The figure shows three views and two pictorial views of one solid part (mm, origin at its lowest corner). Answer the questions. A direction names the side the tool comes from. Round coordinates to 2 decimals unless told otherwise and drop trailing zeros. Loops run counter-clockwise (first coordinate to the right, second up) from the corner with the lowest first, then second, coordinate; pieces in that order, holes last. Notation, with made-up numbers: (-30.5, 12) -> (20.5, 12) arc R25 cw to (20.5, 45) -> close; hole circle Ø11 at (16, 30.5). An arc over 180 degrees is marked (long way). Put each result on its own line as item: value.
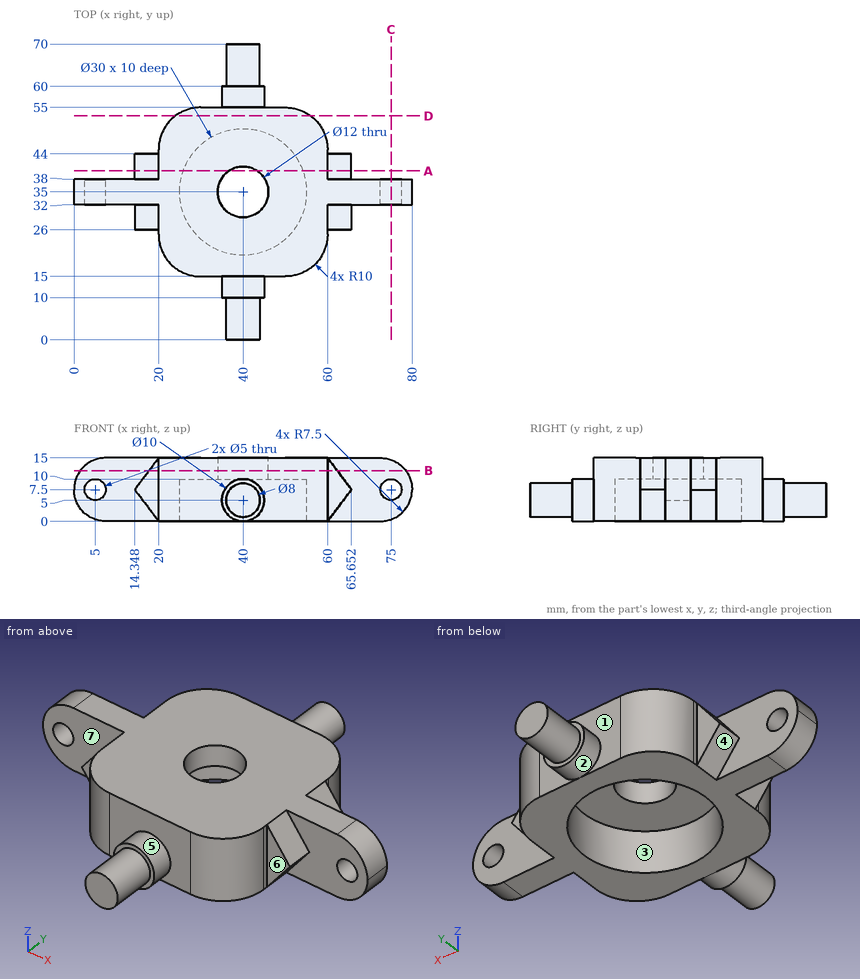
Item 1: The part is cut by section B-B (z = 12). Determine the outline of the cut face in (x, y).
Derived:
outline: (1.5, 32) -> (17.74, 32) -> (17.74, 26) -> (20, 26) -> (20, 25) arc R10 ccw to (30, 15) -> (50, 15) arc R10 ccw to (60, 25) -> (60, 26) -> (62.26, 26) -> (62.26, 32) -> (78.5, 32) -> (78.5, 38) -> (62.26, 38) -> (62.26, 44) -> (60, 44) -> (60, 45) arc R10 ccw to (50, 55) -> (30, 55) arc R10 ccw to (20, 45) -> (20, 44) -> (17.74, 44) -> (17.74, 38) -> (1.5, 38) -> close; hole circle Ø12 at (40, 35)
Item 2: The part is cut by section A-A (y = 40). Determine the outline of the cut face in (x, z).
Derived:
outline: (14.35, 7.5) -> (20, 0) -> (25.86, 0) -> (25.86, 10) -> (36.68, 10) -> (36.68, 15) -> (20, 15) -> close; (43.32, 10) -> (54.14, 10) -> (54.14, 0) -> (60, 0) -> (65.65, 7.5) -> (60, 15) -> (43.32, 15) -> close
Item 3: Which of the six approach directions +Z, -Z, +X, -X, +Y, -Y give full straight-line access (tool end or side, diameter ignored) to the marked faces 4, 5, 6 and 7?
Derived:
face 4: -Z, -X, +Y
face 5: -Y
face 6: +Z, -Z, +X, -Y
face 7: -X, -Y
Item 4: Flat-ended cylindrical pins translate along their axes: pin 1 Ø6 at (x, z) = (47.5, 5.5) entering from -Y; pin 2 Ø5 at (y, z) = (13.5, 9) entering from +X; pin 3 Ø10 at (x, y) = (38, 61) entering from -Z; pin 4 Ø3 at (x, z) = (18, 11) entering from +Y. Find the tip coordinate at first contact, or state that the pin passes through.
Derived:
pin 1: stops at y = 10
pin 2: stops at x = 54.36
pin 3: stops at z = 0
pin 4: stops at y = 44
Item 5: For a pull along Y with two mould halves and no side action, classify the marked faces 1, 2 and 3 as pulls with the +Y half, pulls with the -Y half, needs draft (parallel to the pull), parting line crosses it, or undercut.
Derived:
face 1: pulls with the +Y half
face 2: needs draft
face 3: undercut
Item 6: The part is cut by section D-D (y = 53). Determine the outline of the cut face in (x, z), then the cut area to 3 significant figures.
Derived:
outline: (24, 0) -> (56, 0) -> (56, 15) -> (24, 15) -> close
area: 480 mm^2
Item 7: Find the intervals of material crossed by line 1 along X through (y, z) = (35.4, 7.5) (1 decimal); line 2 along Y through (x, z) = (40, 8.25); line 3 along Y through (x, z) = (17.5, 1.5), in increasing order.
Derived:
line 1: x = 0 to 2.5, 7.5 to 25, 55 to 72.5, 77.5 to 80
line 2: y = 0 to 20, 50 to 70
line 3: y = 32 to 38
Item 8: The part is cut by section C-C (x = 75). Determine the outline of the cut face in (y, z).
Derived:
outline: (32, 0.43) -> (38, 0.43) -> (38, 5) -> (32, 5) -> close; (32, 10) -> (38, 10) -> (38, 14.57) -> (32, 14.57) -> close
